Design review of the part built by this model. Coordinates are the model's own, in mm. Face numbers are marked on the shaded views. A direction names the side the tool comes from. Coordinates: 2 decimals unless noted, no trailing zeros. Loops run counter-clockwise (first coordinate to the right, second up) from the corner with the lowest first, then second, coordinate; pieces in that order, holes last. Notation, with made-up numbers: (-26.75, 24.5) -> (14.25, 24.5) arc R11 cw to (14.25, 35.5) -> close; hole circle Ø10 at (20.5, 33). An arc over 180 degrees is marked (long way). Use one line per item in the form item = value. Start each with the question number.
1. Consider section A-A (x = 38.5). State the section outline as (y, z) points.
2. Machinability: for the marked faces 1, 2 and 3, which of the approach directions +Z, -Z, +X, -X, +Y, -Y give a long, thin tool a straight path to every point of the face, cutting with its end or side? Answer none if there is none.
3. The part is to be moulded in two halves that separate along X. For the marked faces 4, 5 and 6, say which applies: released by +X, released by -X, zero draft, split by the parting line, or undercut.
4. For pin 1 (11 mm diameter, centred on x = 9.89, z = 9.89, fed in from +Y); pin 2 (4.5 mm diameter, centred on x = 38.5, z = -3.75, fed in from +Y); pin 3 (0.6 mm diameter, centred on y = 1, z = 23, fed in from +X), all flat-tipped, find the tip position at first contact; note any pin that passes through.
5. Consider section B-B (z = 13.5). State the section outline as (x, y) points, then the cut area to 3 significant figures.
6. Consider section C-C (y = 31.5). State how many separate pieces and enclosed holes the cut face has, then the cut area to 3 significant figures.
7. Wall thickness on line 1 (Y direction, x = 24, z = 19); line 2 (X direction, y = 0.5, z = 23.75); line 3 (Y direction, x = 16, z = 7): over which ranges is each line inside the solid? List them lowest first. Write a range as from..to.
8. Consider section D-D (y = 5). State the section outline as (x, z) points, then the cut area to 3 significant figures.
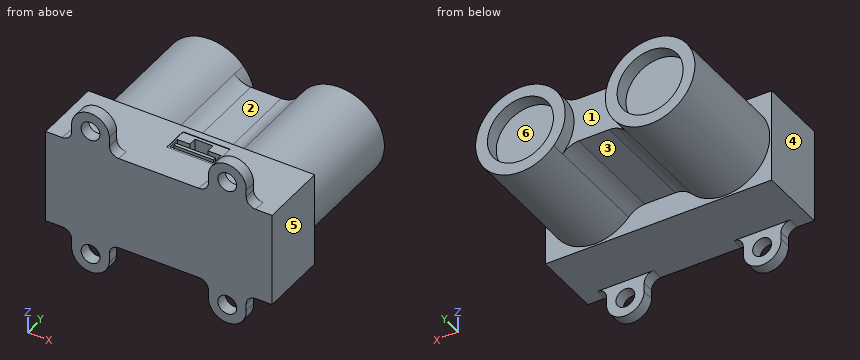
from build123d import *

# Parameters (mm, degrees)
ESQUISSE1_W                 = 48
ESQUISSE1_H                 = 20
BOSS_EXTRU_2_DEPTH          = 40
ESQUISSE1_3_R               = 2
BOSS_EXTRU_4_DEPTH          = 2.5
CONG_1_R                    = 2
ENL_V_START                 = -25.5
ENL_V_MAT_EXTRU_2_OUTLINE_W = 48
ENL_V_MAT_EXTRU_2_OUTLINE_H = 20
ENL_V_MAT_EXTRU_2_DEPTH     = 25.5
ENL_V_START_2               = -3
ENL_V_MAT_EXTRU_3_DEPTH     = 3
ESQUISSE3_5_R               = 7
ENL_V_MAT_EXTRU_4_DEPTH     = 25.5
ESQUISSE8_R                 = 7
BOSS_EXTRU_5_DEPTH          = 2
ESQUISSE9_W                 = 3.806741441
ESQUISSE9_H                 = 1.749254543
ENL_V_MAT_EXTRU_5_DEPTH     = 4
ESQUISSE9_3_W               = 9.246461273
ESQUISSE9_3_H               = 2.546264857
ESQUISSE9_3_W_2             = 8.356621676
ESQUISSE9_3_H_2             = 0.706512752
ENL_V_MAT_EXTRU_6_DEPTH     = 4
ESQUISSE9_5_W               = 10
ESQUISSE9_5_H               = 5.5
ENL_V_MAT_EXTRU_7_DEPTH     = 0.1


# Read off the part's stored shape, not the designer's step: Enlèv. mat.-Extru.2, Enlèv. mat.-Extru.3
with BuildPart() as part:
    # Esquisse1 → Boss.-Extru.2 (new body)
    with BuildSketch(Plane(origin=(0, 0, 0), x_dir=(1, 0, 0), z_dir=(0, 1, 0))):
        with Locations((24, -10)):
            Rectangle(ESQUISSE1_W, ESQUISSE1_H)
    extrude(amount=BOSS_EXTRU_2_DEPTH)

    # Esquisse1<3> → Boss.-Extru.4 (add)
    # profile 1 of 4: a face of its own
    with BuildSketch(Plane(origin=(0, 0, 0), x_dir=(1, 0, 0), z_dir=(0, 1, 0))):
        with BuildLine():
            Line((13.5, -20), (5.5, -20))
            Line((5.5, -20), (5.5, -23.5))
            ThreePointArc((5.5, -23.5), (9.25, -27.75), (13.5, -24))
            Line((13.5, -24), (13.5, -20))
        make_face()
        with Locations(Location((9.5, -23.75, 0), (0, 0, 270))):
            Circle(ESQUISSE1_3_R, mode=Mode.SUBTRACT)
    # profile 2 of 4: a face of its own
    with BuildSketch(Plane(origin=(0, 0, 0), x_dir=(1, 0, 0), z_dir=(0, 1, 0))):
        with BuildLine():
            Line((42.5, -20), (34.5, -20))
            Line((34.5, -20), (34.5, -24))
            ThreePointArc((34.5, -24), (38.75, -27.75), (42.5, -23.5))
            Line((42.5, -23.5), (42.5, -20))
        make_face()
        with Locations(Location((38.5, -23.75, 0), (0, 0, 270))):
            Circle(ESQUISSE1_3_R, mode=Mode.SUBTRACT)
    # profile 3 of 4: a face of its own
    with BuildSketch(Plane(origin=(0, 0, 0), x_dir=(1, 0, 0), z_dir=(0, 1, 0))):
        with BuildLine():
            Line((5.5, 3.5), (5.5, 0))
            Line((5.5, 0), (13.5, 0))
            Line((13.5, 0), (13.5, 4))
            ThreePointArc((13.5, 4), (9.25, 7.75), (5.5, 3.5))
        make_face()
        with Locations(Location((9.5, 3.75, 0), (0, 0, 270))):
            Circle(ESQUISSE1_3_R, mode=Mode.SUBTRACT)
    # profile 4 of 4: a face of its own
    with BuildSketch(Plane(origin=(0, 0, 0), x_dir=(1, 0, 0), z_dir=(0, 1, 0))):
        with BuildLine():
            Line((34.5, 4), (34.5, 0))
            Line((34.5, 0), (42.5, 0))
            Line((42.5, 0), (42.5, 3.5))
            ThreePointArc((42.5, 3.5), (38.75, 7.75), (34.5, 4))
        make_face()
        with Locations(Location((38.5, 3.75, 0), (0, 0, 270))):
            Circle(ESQUISSE1_3_R, mode=Mode.SUBTRACT)
    extrude(amount=BOSS_EXTRU_4_DEPTH)

    # Congé1
    cong_1_edges = [part.edges().sort_by_distance(p)[0] for p in [
        (42.5, 1.25, 0),
        (34.5, 1.25, 0),
        (13.5, 1.25, 0),
        (5.5, 1.25, 0),
        (34.5, 1.25, 20),
        (42.5, 1.25, 20),
        (13.5, 1.25, 20),
        (5.5, 1.25, 20),
    ]]
    fillet(cong_1_edges, radius=CONG_1_R)

    # Enlèv. mat.-Extru.2 outline → Enlèv. mat.-Extru.2 (cut)
    with BuildSketch(Plane(origin=(0, 40, 0), x_dir=(1, 0, 0), z_dir=(0, 1, 0)).offset(ENL_V_START)):
        with Locations((24, -10)):
            Rectangle(ENL_V_MAT_EXTRU_2_OUTLINE_W, ENL_V_MAT_EXTRU_2_OUTLINE_H)
        with BuildLine():
            add(Edge.make_bspline(
                [(16.963589169, -16.237376104), (17.999093762, -15.180393065), (19.150056624, -14.648292989), (20.416477791, -14.641075876)],
                knots=[0, 0, 0, 0, 0.986436325, 0.986436325, 0.986436325, 0.986436325], degree=3))
            ThreePointArc((16.963589169, -16.237376104), (0.394326585, -9.891075881), (16.963589169, -3.544775658))
            add(Edge.make_bspline(
                [(16.963589169, -3.544775658), (17.999093762, -4.601758697), (19.150056624, -5.133858773), (20.416477791, -5.141075886)],
                knots=[0, 0, 0, 0, 0.986436325, 0.986436325, 0.986436325, 0.986436325], degree=3))
            Line((20.416477791, -5.141075886), (26.872175379, -5.141075886))
            add(Edge.make_bspline(
                [(30.325064001, -3.544775658), (29.289559409, -4.601758697), (28.138596547, -5.133858773), (26.872175379, -5.141075886)],
                knots=[0, 0, 0, 0, 0.986436325, 0.986436325, 0.986436325, 0.986436325], degree=3))
            ThreePointArc((30.325064001, -3.544775658), (46.894326585, -9.891075881), (30.325064001, -16.237376104))
            add(Edge.make_bspline(
                [(30.325064001, -16.237376104), (29.289559409, -15.180393065), (28.138596547, -14.648292989), (26.872175379, -14.641075876)],
                knots=[0, 0, 0, 0, 0.986436325, 0.986436325, 0.986436325, 0.986436325], degree=3))
            Line((26.872175379, -14.641075876), (20.416477791, -14.641075876))
        make_face(mode=Mode.SUBTRACT)
    extrude(amount=ENL_V_MAT_EXTRU_2_DEPTH, mode=Mode.SUBTRACT)

    # Enlèv. mat.-Extru.3 outline → Enlèv. mat.-Extru.3 (cut)
    with BuildSketch(Plane(origin=(0, 40, 0), x_dir=(1, 0, 0), z_dir=(0, 1, 0)).offset(ENL_V_START_2)):
        with BuildLine():
            ThreePointArc((30.325064001, -16.237376104), (27.894326585, -9.891075881), (30.325064001, -3.544775658))
            add(Edge.make_bspline(
                [(30.325064001, -3.544775658), (29.289559409, -4.601758697), (28.138596547, -5.133858773), (26.872175379, -5.141075886)],
                knots=[0, 0, 0, 0, 0.986436325, 0.986436325, 0.986436325, 0.986436325], degree=3))
            Line((26.872175379, -5.141075886), (20.416477791, -5.141075886))
            add(Edge.make_bspline(
                [(16.963589169, -3.544775658), (17.999093762, -4.601758697), (19.150056624, -5.133858773), (20.416477791, -5.141075886)],
                knots=[0, 0, 0, 0, 0.986436325, 0.986436325, 0.986436325, 0.986436325], degree=3))
            ThreePointArc((16.963589169, -3.544775658), (19.394326585, -9.891075881), (16.963589169, -16.237376104))
            add(Edge.make_bspline(
                [(16.963589169, -16.237376104), (17.999093762, -15.180393065), (19.150056624, -14.648292989), (20.416477791, -14.641075876)],
                knots=[0, 0, 0, 0, 0.986436325, 0.986436325, 0.986436325, 0.986436325], degree=3))
            Line((20.416477791, -14.641075876), (26.872175379, -14.641075876))
            add(Edge.make_bspline(
                [(30.325064001, -16.237376104), (29.289559409, -15.180393065), (28.138596547, -14.648292989), (26.872175379, -14.641075876)],
                knots=[0, 0, 0, 0, 0.986436325, 0.986436325, 0.986436325, 0.986436325], degree=3))
        make_face()
    extrude(amount=ENL_V_MAT_EXTRU_3_DEPTH, mode=Mode.SUBTRACT)

    # Esquisse3<5> → Enlèv. mat.-Extru.4 (cut)
    with BuildSketch(Plane(origin=(0, 40, 0), x_dir=(1, 0, 0), z_dir=(0, 1, 0))):
        with Locations(Location((9.894326585, -9.891075881, 0), (0, 0, 270))):
            Circle(ESQUISSE3_5_R)
        with Locations(Location((37.394326585, -9.891075881, 0), (0, 0, 270))):
            Circle(ESQUISSE3_5_R)
    extrude(amount=-ENL_V_MAT_EXTRU_4_DEPTH, mode=Mode.SUBTRACT)

    # Esquisse8 → Boss.-Extru.5 (add)
    with BuildSketch(Plane(origin=(0, 37, 0), x_dir=(1, 0, 0), z_dir=(0, 1, 0))):
        with Locations(Location((9.894326585, -9.891075881, 0), (0, 0, 270))):
            Circle(ESQUISSE8_R)
        with Locations(Location((37.394326585, -9.891075881, 0), (0, 0, 270))):
            Circle(ESQUISSE8_R)
    extrude(amount=-BOSS_EXTRU_5_DEPTH)

    # Esquisse9 → Enlèv. mat.-Extru.5 (cut)
    with BuildSketch(Plane.XY.offset(20)):
        with Locations((25.870972193, 11.450343865)):
            Rectangle(ESQUISSE9_W, ESQUISSE9_H)
    extrude(amount=-ENL_V_MAT_EXTRU_5_DEPTH, mode=Mode.SUBTRACT)

    # Esquisse9<3> → Enlèv. mat.-Extru.6 (cut)
    with BuildSketch(Plane.XY.offset(20)):
        with Locations((25.968514368, 9.302584165)):
            Rectangle(ESQUISSE9_3_W, ESQUISSE9_3_H)
        with Locations((25.880686529, 9.127251066)):
            Rectangle(ESQUISSE9_3_W_2, ESQUISSE9_3_H_2, mode=Mode.SUBTRACT)
    extrude(amount=-ENL_V_MAT_EXTRU_6_DEPTH, mode=Mode.SUBTRACT)

    # Esquisse9<5> → Enlèv. mat.-Extru.7 (cut)
    with BuildSketch(Plane.XY.offset(20)):
        with Locations((26, 10.25)):
            Rectangle(ESQUISSE9_5_W, ESQUISSE9_5_H)
    extrude(amount=-ENL_V_MAT_EXTRU_7_DEPTH, mode=Mode.SUBTRACT)


solid = part.part
Geometry check:
q1.outline = (0, -7.76) -> (2.5, -7.76) -> (2.5, -5.75) -> (0, -5.75) -> close; (0, -1.75) -> (2.5, -1.75) -> (2.5, 0) -> (14.5, 0) -> (14.5, 0.46) -> (40, 0.46) -> (40, 2.98) -> (37, 2.98) -> (37, 16.8) -> (40, 16.8) -> (40, 19.33) -> (14.5, 19.33) -> (14.5, 20) -> (2.5, 20) -> (2.5, 21.75) -> (0, 21.75) -> close; (0, 25.75) -> (2.5, 25.75) -> (2.5, 27.76) -> (0, 27.76) -> close; hole (14.5, 2.98) -> (35, 2.98) -> (35, 16.8) -> (14.5, 16.8) -> close
q2.face_1 = +Y
q2.face_2 = +Z, +Y
q2.face_3 = -Z, +Y
q3.face_4 = released by -X
q3.face_5 = released by +X
q3.face_6 = undercut
q4.pin_1 = 37
q4.pin_2 = 2.5
q4.pin_3 = 42.5
q5.outline = (0, 0) -> (48, 0) -> (48, 14.5) -> (46.18, 14.5) -> (46.18, 40) -> (43.39, 40) -> (43.39, 37) -> (31.4, 37) -> (31.4, 40) -> (28.61, 40) -> (28.61, 37) -> (18.68, 37) -> (18.68, 40) -> (15.89, 40) -> (15.89, 37) -> (3.9, 37) -> (3.9, 40) -> (1.11, 40) -> (1.11, 14.5) -> (0, 14.5) -> close; hole (3.9, 14.5) -> (15.89, 14.5) -> (15.89, 35) -> (3.9, 35) -> close; hole (31.4, 14.5) -> (43.39, 14.5) -> (43.39, 35) -> (31.4, 35) -> close
q5.area = 1,250 mm²
q6.separate_pieces = 1
q6.enclosed_holes = 2
q6.area = 351 mm²
q7.line_1 = 0..8.03, 8.77..9.48, 12.32..14.5
q7.line_2 = 5.49..7.5, 11.5..13.5, 34.5..36.5, 40.5..42.51
q7.line_3 = 0..14.5, 35..37
q8.outline = (0, 0) -> (48, 0) -> (48, 20) -> (0, 20) -> close
q8.area = 960 mm²
